Drawing for the job (mm, zero at the part's lowest x, y, z). A direction names the side the tool comes from. Give positions to 0.01 mm unless a question says otherwise; leave off trailing zeros. Loops run counter-clockwise (first coordinate to the right, second up) from the corner with the lowest first, then second, coordinate; pieces in that order, holes last. Notation, with made-up numbers: (-6, 34) -> (5, 34) arc R28 ccw to (5, 64) -> close; hole circle Ø5 at (31.25, 68). An arc over 180 degrees is marked (long way). Answer in a Markdown table with one row per item. Add a question column.
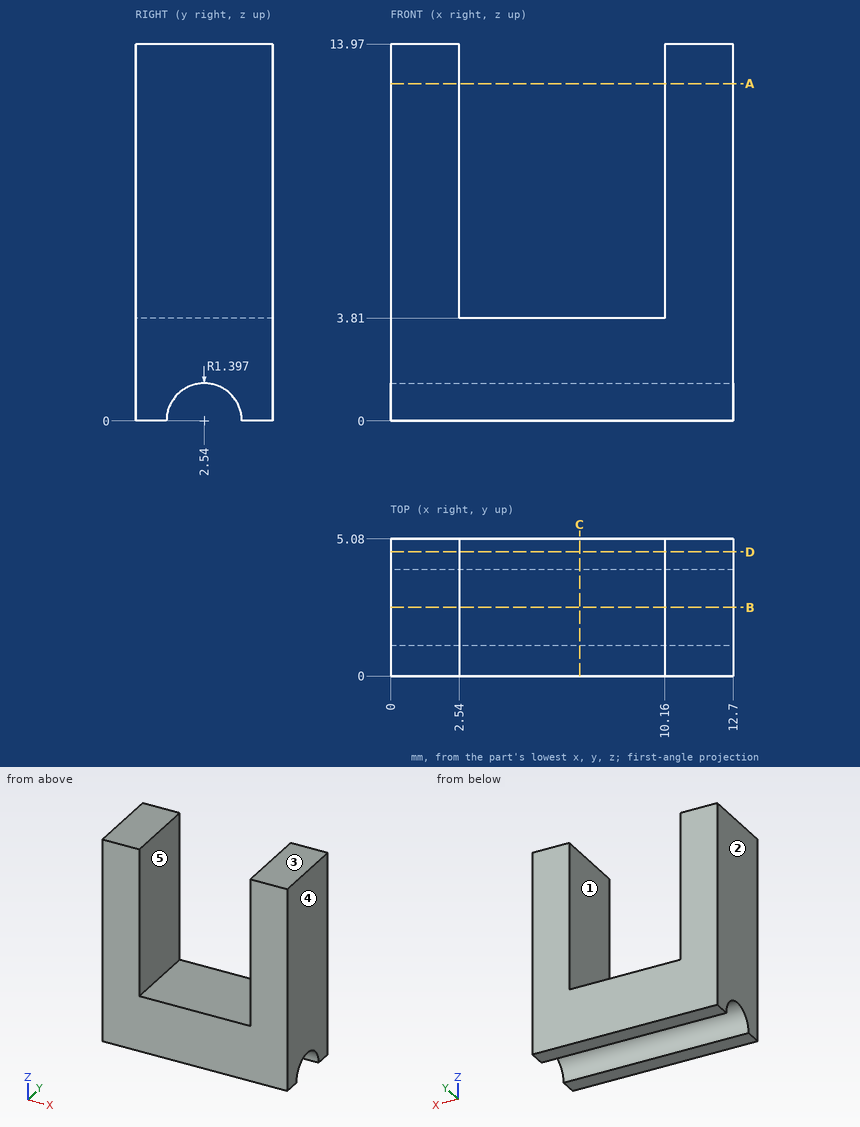
(1) Flat gauge pins, fed straight in: pin 1 Ø3 at (x, y) = (7, 3) entering from +Z; pin 2 Ø1.5 at (x, z) = (8, 8) entering from +Y. Where does each tip first touch, or does it go through?
(2) Saw through at C-C, the plane x = 7. List the corners of the cut face in (y, z), then the cut area to 3 significant figures.
(3) Saw through at D-D, the plane y = 4.6. List the corners of the cut face in (x, z), then the cut area to 4 significant figures.
(4) Saw through at B-B, the plane y = 2.54. List the corners of the cut face in (x, z), then the cut area to 3 significant figures.
(5) Two-plate mould, pull along X, no slides. Class the marked faces 3, 4 and 5: released by +X, released by -X, zero draft, split by the parting line, or undercut.
(6) 3-axis set-ups, long thin cutter, end or side, ignore diameter. For the marked faces 1 and 2: which of +Z, -Z, +X, -X, +Y, -Y reach the whole face in a straight line?
(7) Saw through at A-A, the plane z = 12.5. List the corners of the cut face in (x, y), then the cut area to 3 significant figures.
(8) Wall check: line 1 along X through (y, z) = (3.85, 5); line 2 along Z through (x, y) = (5.5, 4.8); line 3 along Z through (x, y) = (1.75, 3.1). Give the ranges that are in metal, low to high. Write a range as from..to.
Worked answers:
| question | item | result |
|---|---|---|
| 1 | pin 1 | z = 3.81 |
| 1 | pin 2 | through |
| 2 | outline | (0, 0) -> (1.14, 0) arc R1.4 cw to (3.94, 0) -> (5.08, 0) -> (5.08, 3.81) -> (0, 3.81) -> close |
| 2 | area | 16.3 mm^2 |
| 3 | outline | (0, 0) -> (12.7, 0) -> (12.7, 13.97) -> (10.16, 13.97) -> (10.16, 3.81) -> (2.54, 3.81) -> (2.54, 13.97) -> (0, 13.97) -> close |
| 3 | area | 100.0 mm^2 |
| 4 | outline | (0, 1.4) -> (12.7, 1.4) -> (12.7, 13.97) -> (10.16, 13.97) -> (10.16, 3.81) -> (2.54, 3.81) -> (2.54, 13.97) -> (0, 13.97) -> close |
| 4 | area | 82.3 mm^2 |
| 5 | face 3 | zero draft |
| 5 | face 4 | released by +X |
| 5 | face 5 | undercut |
| 6 | face 1 | +Z, +Y, -Y |
| 6 | face 2 | +Z, -Z, -X, +Y, -Y |
| 7 | outline | (0, 0) -> (2.54, 0) -> (2.54, 5.08) -> (0, 5.08) -> close; (10.16, 0) -> (12.7, 0) -> (12.7, 5.08) -> (10.16, 5.08) -> close |
| 7 | area | 25.8 mm^2 |
| 8 | line 1 | 0..2.54, 10.16..12.7 |
| 8 | line 2 | 0..3.81 |
| 8 | line 3 | 1.28..13.97 |
